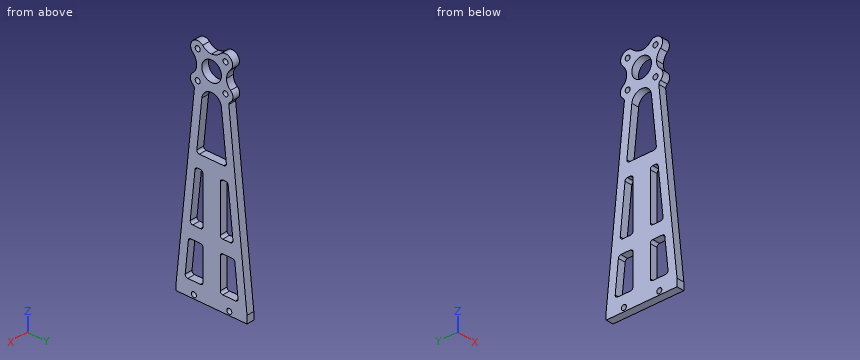
```python
from build123d import *

# Parameters (mm, degrees)
SKETCH1_R            = 6.25
BOSS_EXTRUDE1_DEPTH  = 2.3815
M3_CLEARANCE_HOLE1_D = 3.2
M3_CLEARANCE_HOLE2_D = 3.2


with BuildPart() as part:
    # Sketch1 → Boss-Extrude1 (new body, symmetric)
    with BuildSketch(Plane(origin=(0, 0, 0), x_dir=(0, 0, -1), z_dir=(1, 0, 0))):
        with BuildLine():
            Line((13.837853408, 10.933433942), (125.499999966, 22.5))
            Line((125.499999966, 22.5), (130.262999966, 22.5))
            Line((130.262999966, 22.5), (130.262999966, -22.5))
            Line((130.262999966, -22.5), (125.499999966, -22.5))
            Line((125.499999966, -22.5), (13.842307627, -10.933864535))
            ThreePointArc((13.842307627, -10.933864535), (12.834192522, -11.314170817), (12.02081528, -12.02081528))
            ThreePointArc((12.02081528, -12.02081528), (8.840593, -13.543231212), (5.659233624, -12.023192877))
            ThreePointArc((5.659233624, -12.023192877), (3.133291337, -10.08048914), (0, -9.5))
            ThreePointArc((0, -9.5), (-3.061848318, -10.236700307), (-5.656913672, -12.020874702))
            ThreePointArc((-5.656913672, -12.020874702), (-12.020874702, -12.020874704), (-12.020874704, -5.656913674))
            ThreePointArc((-12.020874704, -5.656913674), (-10.079850186, -3.131745006), (-9.500000034, 0))
            ThreePointArc((-9.500000034, 0), (-10.236707938, 3.061753973), (-12.020757217, 5.656796188))
            ThreePointArc((-12.020757217, 5.656796188), (-12.02045467, 12.020757197), (-5.65649366, 12.02045465))
            ThreePointArc((-5.65649366, 12.02045465), (-3.061652792, 10.236409392), (0, 9.5))
            ThreePointArc((0, 9.5), (3.130793061, 10.079739971), (5.655645869, 12.019606441))
            ThreePointArc((5.655645869, 12.019606441), (8.837941978, 13.539821179), (12.02081528, 12.02081528))
            ThreePointArc((12.02081528, 12.02081528), (12.832791387, 11.315799207), (13.837853408, 10.933433942))
        make_face()
        Circle(SKETCH1_R, mode=Mode.SUBTRACT)
        with BuildLine():
            Line((17.302023212, 6.215300033), (47.183954034, 9.358065674))
            ThreePointArc((47.183954034, 9.358065674), (48.412204848, 8.959051834), (48.9375, 7.779273418))
            Line((48.9375, 7.779273418), (48.9375, -7.779269087))
            ThreePointArc((48.9375, -7.779269087), (48.412206576, -8.959045947), (47.183958659, -9.358061829))
            Line((47.183958659, -9.358061829), (17.302047548, -6.21538676))
            ThreePointArc((17.302047548, -6.21538676), (11.709307369, -5.4312e-05), (17.302023212, 6.215300033))
        make_face(mode=Mode.SUBTRACT)
        with BuildLine():
            Line((57.09375, 8.955806876), (57.09375, 7.0875))
            ThreePointArc((57.09375, 7.0875), (57.558717985, 5.964967985), (58.68125, 5.5))
            Line((58.68125, 5.5), (88.13125, 5.5))
            ThreePointArc((88.13125, 5.5), (89.253782015, 5.964967985), (89.71875, 7.0875))
            Line((89.71875, 7.0875), (89.71875, 12.006396363))
            ThreePointArc((89.71875, 12.006396363), (89.194380816, 13.185340432), (87.967683395, 13.585447412))
            Line((87.967683395, 13.585447412), (58.517683395, 10.534857925))
            ThreePointArc((58.517683395, 10.534857925), (57.502305931, 10.018937692), (57.09375, 8.955806876))
        make_face(mode=Mode.SUBTRACT)
        with BuildLine():
            Line((58.68125, -5.5), (88.13125, -5.5))
            ThreePointArc((88.13125, -5.5), (89.253782015, -5.964967985), (89.71875, -7.0875))
            Line((89.71875, -7.0875), (89.71875, -12.006377313))
            ThreePointArc((89.71875, -12.006377313), (89.194380958, -13.185321253), (87.967683776, -13.585428401))
            Line((87.967683776, -13.585428401), (58.517683776, -10.534846102))
            ThreePointArc((58.517683776, -10.534846102), (57.502306059, -10.018925972), (57.09375, -8.955795013))
            Line((57.09375, -8.955795013), (57.09375, -7.0875))
            ThreePointArc((57.09375, -7.0875), (57.558717985, -5.964967985), (58.68125, -5.5))
        make_face(mode=Mode.SUBTRACT)
        with BuildLine():
            Line((99.298933395, 14.759199267), (118.74893336, 16.773934935))
            ThreePointArc((118.74893336, 16.773934935), (119.975630782, 16.373827955), (120.499999966, 15.194883886))
            Line((120.499999966, 15.194883886), (120.499999966, 7.0875))
            ThreePointArc((120.499999966, 7.0875), (120.035031981, 5.964967985), (118.912499966, 5.5))
            Line((118.912499966, 5.5), (99.4625, 5.5))
            ThreePointArc((99.4625, 5.5), (98.339967985, 5.964967985), (97.875, 7.0875))
            Line((97.875, 7.0875), (97.875, 13.180148218))
            ThreePointArc((97.875, 13.180148218), (98.283555931, 14.243279034), (99.298933395, 14.759199267))
        make_face(mode=Mode.SUBTRACT)
        with BuildLine():
            Line((118.912499966, -5.5), (99.4625, -5.5))
            ThreePointArc((99.4625, -5.5), (98.339967985, -5.964967985), (97.875, -7.0875))
            Line((97.875, -7.0875), (97.875, -13.180126402))
            ThreePointArc((97.875, -13.180126402), (98.283556059, -14.24325736), (99.298933776, -14.759177491))
            Line((99.298933776, -14.759177491), (118.748933742, -16.773908412))
            ThreePointArc((118.748933742, -16.773908412), (119.975630924, -16.373801264), (120.499999966, -15.194857323))
            Line((120.499999966, -15.194857323), (120.499999966, -7.0875))
            ThreePointArc((120.499999966, -7.0875), (120.035031981, -5.964967985), (118.912499966, -5.5))
        make_face(mode=Mode.SUBTRACT)
    extrude(amount=BOSS_EXTRUDE1_DEPTH, both=True)

    # M3 Clearance Hole1 (through all)
    with Locations(Plane(origin=(2.3815, 0, 0), x_dir=(0, 0, -1), z_dir=(1, 0, 0))):
        with Locations((127.881499966, 11.25), (127.881499966, -11.25)):
            Hole(M3_CLEARANCE_HOLE1_D / 2)

    # M3 Clearance Hole2 (through all)
    with Locations(Plane(origin=(2.3815, 0, 0), x_dir=(0, 0, -1), z_dir=(1, 0, 0))):
        with Locations((-8.838834765, 8.838834765), (8.838834765, 8.838834765), (8.838834765, -8.838834765), (-8.838834765, -8.838834765)):
            Hole(M3_CLEARANCE_HOLE2_D / 2)


solid = part.part
```
The listing builds one solid part. Answer for the finished solid, in the listing's coordinates (mm). Coordinates: 2 decimals unless noted, no trailing zeros. Write each loop counter-clockwise with the first axis right and the second up, starting at its lowest first coordinate (ties: lowest second). Pieces come first, ordered by that corner, then holes. Notation, with made-up numbers: (2.25, 6.25) -> (20.25, 6.25) arc R21 cw to (20.25, 36.25) -> close; hole circle Ø11 at (-34, 67.25). An arc over 180 degrees is marked (long way). Write each question's results on one line, items separated by ' | '. Start each with the question number.
1) A cutting plane is placed at A-A (z = -111.5). Determine the outline of the cut face in (x, y).
2) Straight lines are drawn through the part: probe 1 along Y at (x, z) = (1.8, -117); probe 2 along Y at (x, z) = (0.3, -111.5); probe 3 along Y at (x, z) = (-1.7, -0.5). For each, find the intervals that lie inside material, in ascending order.
3) A cutting plane is placed at B-B (z = -29). Determine the outline of the cut face in (x, y), then the cut area to 3 significant figures.
4) Flat-ended cylindrical pins translate along their axes: pin 1 Ø1.5 at (x, y) = (2, -11.5) entering from +Z; pin 2 Ø1.4 at (x, y) = (0, -0.5) entering from +Z; pin 3 Ø12 at (y, z) = (10, -77.5) entering from +X; pin 4 Ø2 at (x, z) = (0.5, -49) entering from -Y. Find the tip coordinate at first contact, or state that the pin passes through.
5) A cutting plane is placed at D-D (z = 3.5). Determine the outline of the cut face in (x, y), then the cut area to 3 significant figures.
6) A cutting plane is placed at C-C (x = 1.05). Count the separate pieces of the cut face and the enclosed holes in it, then the cut area to 3 significant figures.
Values follow:
1) outline: (-2.38, -21.05) -> (2.38, -21.05) -> (2.38, -16.02) -> (-2.38, -16.02) -> close; (-2.38, -5.5) -> (2.38, -5.5) -> (2.38, 5.5) -> (-2.38, 5.5) -> close; (-2.38, 16.02) -> (2.38, 16.02) -> (2.38, 21.05) -> (-2.38, 21.05) -> close
2) probe 1: -21.62 to -16.59, -5.5 to 5.5, 16.59 to 21.62 | probe 2: -21.05 to -16.02, -5.5 to 5.5, 16.02 to 21.05 | probe 3: -9.49 to -6.23, 6.23 to 9.49
3) outline: (-2.38, -12.5) -> (2.38, -12.5) -> (2.38, -7.45) -> (-2.38, -7.45) -> close; (-2.38, 7.45) -> (2.38, 7.45) -> (2.38, 12.5) -> (-2.38, 12.5) -> close | area: 48.2 mm²
4) pin 1: z = 12.91 | pin 2: z = 9.54 | pin 3: x = 2.38 | pin 4: y = -14.68
5) outline: (-2.38, -10.45) -> (2.38, -10.45) -> (2.38, -5.18) -> (-2.38, -5.18) -> close; (-2.38, 5.18) -> (2.38, 5.18) -> (2.38, 10.45) -> (-2.38, 10.45) -> close | area: 50.2 mm²
6) separate pieces: 1 | enclosed holes: 12 | area: 2,940 mm²
